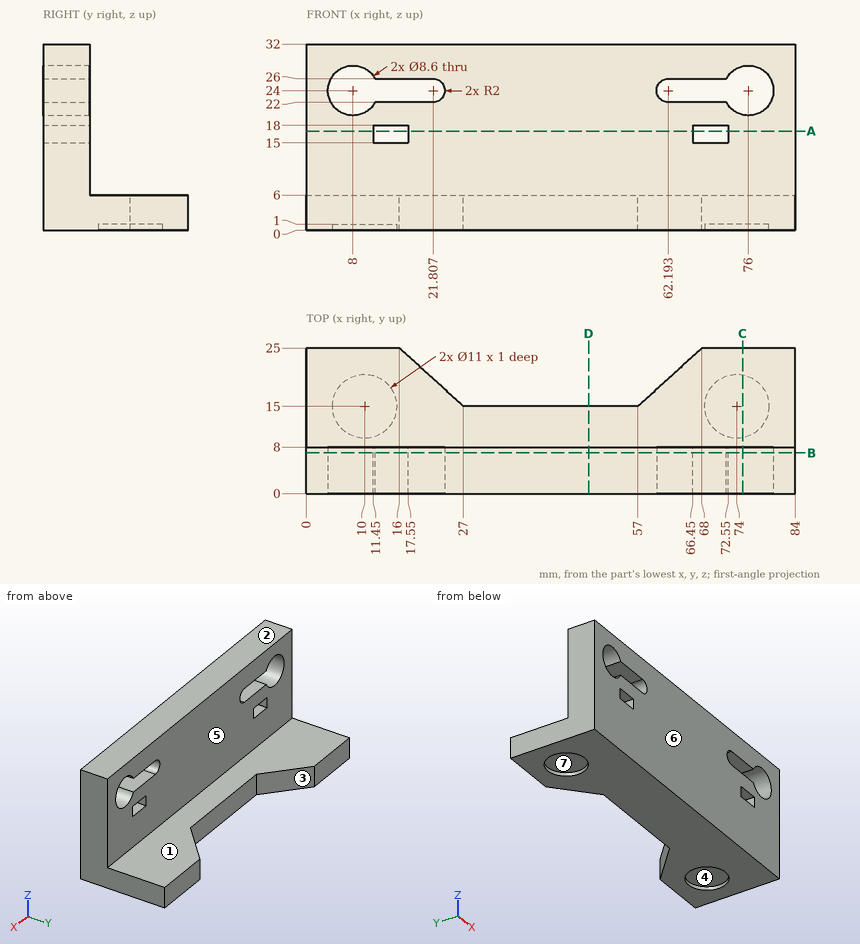
Study the drawing (mm; zero at the part's minimum x, y, z) and answer. A direction names the side the tool comes from. Round coordinates to 2 decimals unless told otherwise and drop trailing zeros. Write each loop counter-clockwise with the first axis right and the second up, starting at its lowest first coordinate (ties: lowest second). Pieces come first, ordered by that corner, then holes. Notation, with made-up numbers: (40.25, -32.75) -> (44.25, -32.75) arc R24 cw to (44.25, -19.75) -> close; hole circle Ø2 at (32.25, 80.25). An arc over 180 degrees is marked (long way). Write item = value, one per line.
1) Which of the six approach directions +Z, -Z, +X, -X, +Y, -Y give full straight-line access (tool end or side, diameter ignored) to the marked faces 1, 2 and 3?
Check values:
face_1 = +Z, +X, -X, +Y
face_2 = +Z, +X, -X, +Y, -Y
face_3 = +Z, -Z, +Y
2) Section D-D on x = 48.5 is taken. Write down the section's boundary in (y, z), plus the area to 3 significant figures.
Check values:
outline = (0, 0) -> (15, 0) -> (15, 6) -> (8, 6) -> (8, 32) -> (0, 32) -> close
area = 298 mm²
3) Section A-A on z = 17 is taken. Write down the section's boundary in (x, y).
Check values:
outline = (0, 0) -> (11.45, 0) -> (11.45, 8) -> (0, 8) -> close; (17.55, 0) -> (66.45, 0) -> (66.45, 8) -> (17.55, 8) -> close; (72.55, 0) -> (84, 0) -> (84, 8) -> (72.55, 8) -> close
4) Section B-B on y = 7 is taken. Write down the section's boundary in (x, z), plus the area to 3 significant figures.
Check values:
outline = (0, 0) -> (84, 0) -> (84, 32) -> (0, 32) -> close; hole (11.45, 15) -> (17.55, 15) -> (17.55, 18) -> (11.45, 18) -> close; hole (11.81, 22) -> (21.81, 22) arc R2 ccw to (21.81, 26) -> (11.81, 26) arc R4.3 ccw (long way) to start; hole (62.19, 22) -> (72.19, 22) arc R4.3 ccw (long way) to (72.19, 26) -> (62.19, 26) arc R2 ccw to start; hole (66.45, 15) -> (72.55, 15) -> (72.55, 18) -> (66.45, 18) -> close
area = 2,450 mm²
5) Given pin 1 (5 mm diameter, centred on x = 35.5, z = 3, fed in from +Y); pin 2 (14 mm diameter, centred on x = 8, z = 24, fed in from +Y); pin 3 (7.5 mm diameter, centred on x = 76, z = 24, fed in from +Y), each flat-ended and moving along its own axis, determine where each tip first touches the part or whether it passes through.
Check values:
pin_1 = 15
pin_2 = 8
pin_3 = through
6) Section C-C on x = 75 is taken. Write down the section's boundary in (y, z), plus the area to 3 significant figures.
Check values:
outline = (0, 0) -> (9.59, 0) -> (9.59, 1) -> (20.41, 1) -> (20.41, 0) -> (25, 0) -> (25, 6) -> (8, 6) -> (8, 19.82) -> (0, 19.82) -> close; (0, 28.18) -> (8, 28.18) -> (8, 32) -> (0, 32) -> close
area = 280 mm²
7) Straight lines are drawn through the part: line 1 along Z through (x, y) = (8, 5.25); line 2 along Y through (x, z) = (10, 0.4); line 3 along Z through (x, y) = (66, 1.75). For each, find the intervals that lie inside material, in ascending order. Write a range as [from, to].
Check values:
line_1 = [0, 19.7], [28.3, 32]
line_2 = [0, 9.5], [20.5, 25]
line_3 = [0, 22], [26, 32]
8) For a pull along Y with two mould halves and no side action, classify the marked faces 4, 5, 6 and 7 as released by +Y, released by -Y, zero draft, split by the parting line, or undercut.
Check values:
face_4 = undercut
face_5 = released by +Y
face_6 = released by -Y
face_7 = undercut
